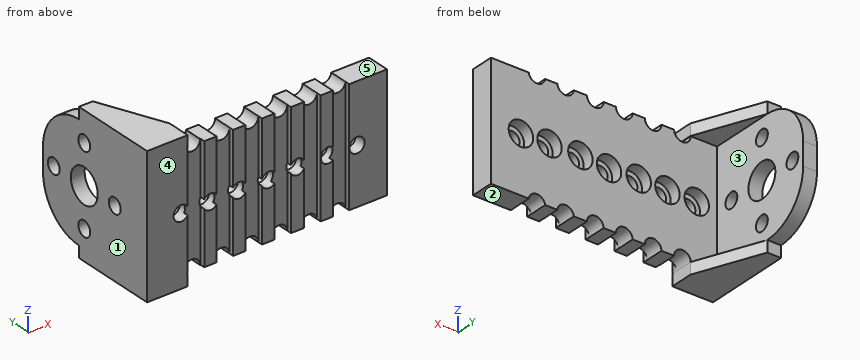
```python
from build123d import *

# Parameters (mm, degrees)
ESBO_O1_W                = 3
ESBO_O1_H                = 25
RESSALTO_EXTRUS_O2_DEPTH = 29
ESBO_O1_4_W              = 49
ESBO_O1_4_H              = 25
RESSALTO_EXTRUS_O3_DEPTH = 5
FILETE2_R                = 10
FILETE3_R                = 10
ESBO_O8_R                = 1.65
CORTE_EXTRUS_O5_DEPTH    = 5
ESBO_O9_R                = 1.8
CORTE_EXTRUS_O6_DEPTH    = 5
ESBO_O10_W               = 3.6
ESBO_O10_H               = 25
ESBO_O10_W_2             = 3.599774239
ESBO_O10_W_3             = 3.58084234
ESBO_O10_W_4             = 3.559844881
CORTE_EXTRUS_O7_DEPTH    = 1
ESBO_O11_R               = 2.65
CORTE_EXTRUS_O8_DEPTH    = 2.5
ESBO_O6_R                = 3.75
ESBO_O6_R_2              = 1.65
CORTE_EXTRUS_O9_DEPTH    = 10
RESSALTO_EXTRUS_O4_DEPTH = 2.5
RESSALTO_EXTRUS_O5_DEPTH = 2.5


with BuildPart() as part:
    # Esbo_o1 → Ressalto-extrus_o2 (new body)
    with BuildSketch(Plane(origin=(0, 0, 0), x_dir=(1, 0, 0), z_dir=(0, 1, 0))):
        with Locations((-24.963414634, 1.243902439)):
            Rectangle(ESBO_O1_W, ESBO_O1_H)
    extrude(amount=RESSALTO_EXTRUS_O2_DEPTH)

    # Esbo_o1_4 → Ressalto-extrus_o3 (add)
    with BuildSketch(Plane(origin=(0, 0, 0), x_dir=(1, 0, 0), z_dir=(0, 1, 0))):
        with Locations((1.036585366, 1.243902439)):
            Rectangle(ESBO_O1_4_W, ESBO_O1_4_H)
    extrude(amount=RESSALTO_EXTRUS_O3_DEPTH)

    # Filete2
    filete2_edges = [part.edges().sort_by_distance(p)[0] for p in [
        (-24.963414634, 29, -13.743902439),
    ]]
    fillet(filete2_edges, radius=FILETE2_R)

    # Filete3
    filete3_edges = [part.edges().sort_by_distance(p)[0] for p in [
        (-24.963414634, 29, 11.256097561),
    ]]
    fillet(filete3_edges, radius=FILETE3_R)

    # Esbo_o8 → Corte-extrus_o5 (cut)
    with BuildSketch(Plane(origin=(0, 5, 0), x_dir=(1, 0, 0), z_dir=(0, 1, 0))):
        with Locations(Location((-19.063414634, 1.243902439, 0), (0, 0, 270))):
            Circle(ESBO_O8_R)
        with Locations(Location((-12.713414634, 1.243902439, 0), (0, 0, 270))):
            Circle(ESBO_O8_R)
        with Locations(Location((-6.497326215, 1.203335799, 0), (0, 0, 270))):
            Circle(ESBO_O8_R)
        with Locations(Location((-0.050914634, 1.451274706, 0), (0, 0, 270))):
            Circle(ESBO_O8_R)
        with Locations(Location((6.147558039, 1.120689497, 0), (0, 0, 270))):
            Circle(ESBO_O8_R)
        with Locations(Location((12.841908527, 1.203335799, 0), (0, 0, 270))):
            Circle(ESBO_O8_R)
        with Locations(Location((19.040381201, 1.451274706, 0), (0, 0, 270))):
            Circle(ESBO_O8_R)
    extrude(amount=-CORTE_EXTRUS_O5_DEPTH, mode=Mode.SUBTRACT)

    # Esbo_o9 → Corte-extrus_o6 (cut)
    with BuildSketch(Plane.XZ):
        with Locations((-15.963414634, 11.256097561)):
            Circle(ESBO_O9_R)
        with Locations((-9.613414634, 11.256097561)):
            Circle(ESBO_O9_R)
        with Locations((-3.356766727, 11.27625585)):
            Circle(ESBO_O9_R)
        with Locations((2.924352249, 11.27625585)):
            Circle(ESBO_O9_R)
        with Locations((9.37076383, 11.441548455)):
            Circle(ESBO_O9_R)
        with Locations((15.569236503, 11.524194757)):
            Circle(ESBO_O9_R)
        with Locations((15.569236503, -14.011999635)):
            Circle(ESBO_O9_R)
        with Locations((9.37076383, -13.929353333)):
            Circle(ESBO_O9_R)
        with Locations((2.924352249, -13.764060728)):
            Circle(ESBO_O9_R)
        with Locations((-3.356766727, -13.764060728)):
            Circle(ESBO_O9_R)
        with Locations((-9.613414634, -13.743902439)):
            Circle(ESBO_O9_R)
        with Locations((-15.963414634, -13.743902439)):
            Circle(ESBO_O9_R)
    extrude(amount=-CORTE_EXTRUS_O6_DEPTH, mode=Mode.SUBTRACT)

    # Esbo_o10 → Corte-extrus_o7 (cut)
    with BuildSketch(Plane.XZ):
        with Locations((-15.863414634, -1.243902439)):
            Rectangle(ESBO_O10_W, ESBO_O10_H)
        with Locations((-9.613414634, -1.243902439)):
            Rectangle(ESBO_O10_W, ESBO_O10_H)
        with Locations((-3.356766727, -1.243902439)):
            Rectangle(ESBO_O10_W_2, ESBO_O10_H)
        with Locations((2.92435225, -1.243902439)):
            Rectangle(ESBO_O10_W_2, ESBO_O10_H)
        with Locations((9.37076383, -1.243902439)):
            Rectangle(ESBO_O10_W_3, ESBO_O10_H)
        with Locations((15.569236504, -1.243902439)):
            Rectangle(ESBO_O10_W_4, ESBO_O10_H)
    extrude(amount=-CORTE_EXTRUS_O7_DEPTH, mode=Mode.SUBTRACT)

    # Esbo_o11 → Corte-extrus_o8 (cut)
    with BuildSketch(Plane(origin=(0, 5, 0), x_dir=(1, 0, 0), z_dir=(0, 1, 0))):
        with Locations(Location((-19.063414634, 1.243902439, 0), (0, 0, 270))):
            Circle(ESBO_O11_R)
        with Locations(Location((-12.713414634, 1.243902439, 0), (0, 0, 270))):
            Circle(ESBO_O11_R)
        with Locations(Location((-6.497326215, 1.203335799, 0), (0, 0, 270))):
            Circle(ESBO_O11_R)
        with Locations(Location((-0.050914634, 1.451274706, 0), (0, 0, 270))):
            Circle(ESBO_O11_R)
        with Locations(Location((6.147558039, 1.120689497, 0), (0, 0, 270))):
            Circle(ESBO_O11_R)
        with Locations(Location((12.841908527, 1.203335799, 0), (0, 0, 270))):
            Circle(ESBO_O11_R)
        with Locations(Location((19.040381201, 1.451274706, 0), (0, 0, 270))):
            Circle(ESBO_O11_R)
    extrude(amount=-CORTE_EXTRUS_O8_DEPTH, mode=Mode.SUBTRACT)

    # Esbo_o6 → Corte-extrus_o9 (cut)
    with BuildSketch(Plane(origin=(-23.463414634, 0, 0), x_dir=(0, 0, -1), z_dir=(1, 0, 0))):
        with Locations((1.243902439, 17.5)):
            Circle(ESBO_O6_R)
        with Locations((9.743902439, 17.5)):
            Circle(ESBO_O6_R_2)
        with Locations((-7.256097561, 17.5)):
            Circle(ESBO_O6_R_2)
        with Locations((1.243902439, 26)):
            Circle(ESBO_O6_R_2)
        with Locations((1.243902439, 9)):
            Circle(ESBO_O6_R_2)
    extrude(amount=-CORTE_EXTRUS_O9_DEPTH, mode=Mode.SUBTRACT)

    # Esbo_o29 → Ressalto-extrus_o4 (add)
    with BuildSketch(Plane.XY.offset(11.256097561)):
        Polygon((-23.463414634, 19), (-17.663414634, 5), (-17.663414634, 0), (-26.463414634, 0), (-26.463414634, 19), align=None)
    extrude(amount=RESSALTO_EXTRUS_O4_DEPTH)

    # Esbo_o30 → Ressalto-extrus_o5 (add)
    with BuildSketch(Plane(origin=(0, 0, -13.743902439), x_dir=(-1, 0, 0), z_dir=(0, 0, -1))):
        Polygon((23.463414634, 19), (17.663414634, 5), (17.663414634, 0), (26.463414634, 0), (26.463414634, 19), align=None)
    extrude(amount=RESSALTO_EXTRUS_O5_DEPTH)


solid = part.part
```
Input: part model. Units: mm. Frame: model coordinates. Face numbers are marked on the shaded views. A direction names the side the tool comes from. Round coordinates to 2 decimals unless told otherwise and drop trailing zeros. Loops run counter-clockwise (first coordinate to the right, second up) from the corner with the lowest first, then second, coordinate; pieces in that order, holes last. Notation, with made-up numbers: (-25, 55) -> (14, 55) arc R36 cw to (14, 89) -> close; hole circle Ø2 at (-3.75, 87). An arc over 180 degrees is marked (long way). Use one line per item in the form item = value. Start each with the question number.
Item 1: Contact query for flat-ended pins moving along their axis: pin 1 Ø1.1 at (x, z) = (-10.5, -2.5) entering from -Y; pin 2 Ø1.3 at (x, y) = (0, 3.5) entering from -Z; pin 3 Ø4 at (x, z) = (6.5, -2.5) entering from +Y. Output: stop coordinate, or through.
Item 2: Section query B-B on y = 26. Return the cut outline in (x, z).
Item 3: Mould query, pull axis Z, two halves, no side actions, for the marked faces 3, 4 and 5. Classes: pulls with the +Z half, pulls with the -Z half, needs draft (parallel to the pull), parting line crosses it, or undercut.
Item 4: Section query D-D on y = 17.5. Return the cut outline in (x, z).
Item 5: Section query A-A on x = -20. Return the cut outline in (y, z), then the cut area to 3 significant figures.
Item 6: Material intervals for L1, parallel to Y at x = -1, z = -12; L2, parallel to X at y = 21.5, z = -7; L3, parallel to Y at x = -16, z = -9.5, sorted ascending. Write a range as from..to.
Item 7: Set-up query: the marked faces 1 and 2. Return all of +Z, -Z, +X, -X, +Y, -Y with unobstructed straight access to the full face (end or side cutting, diameter ignored); none if empty.
Ans:
q1.pin_1 = 1
q1.pin_2 = -13.74
q1.pin_3 = 5
q2.outline = (-26.46, -10.89) -> (-23.46, -10.89) -> (-23.46, -2.89) -> (-26.46, -2.89) -> close; (-26.46, 0.41) -> (-23.46, 0.41) -> (-23.46, 8.4) -> (-26.46, 8.4) -> close
q3.face_3 = undercut
q3.face_4 = needs draft
q3.face_5 = pulls with the +Z half
q4.outline = (-26.46, -16.24) -> (-22.84, -16.24) -> (-22.84, -13.74) -> (-23.46, -13.74) -> (-23.46, -11.39) -> (-26.46, -11.39) -> close; (-26.46, -8.09) -> (-23.46, -8.09) -> (-23.46, -4.99) -> (-26.46, -4.99) -> close; (-26.46, 2.51) -> (-23.46, 2.51) -> (-23.46, 5.61) -> (-26.46, 5.61) -> close; (-26.46, 8.91) -> (-23.46, 8.91) -> (-23.46, 11.26) -> (-22.84, 11.26) -> (-22.84, 13.76) -> (-26.46, 13.76) -> close
q5.outline = (0, -16.24) -> (10.64, -16.24) -> (10.64, -13.74) -> (5, -13.74) -> (5, -3.72) -> (2.5, -3.72) -> (2.5, -2.6) -> (0, -2.6) -> close; (0, 0.11) -> (2.5, 0.11) -> (2.5, 1.24) -> (5, 1.24) -> (5, 11.26) -> (10.64, 11.26) -> (10.64, 13.76) -> (0, 13.76) -> close
q5.area = 159 mm^2
q6.L1 = 0..5
q6.L2 = -26.46..-23.46
q6.L3 = 1..5
q7.face_1 = +Z, -Z, -X, +Y, -Y
q7.face_2 = -Z, +X, +Y, -Y
